from build123d import *
from OCP.BRepFilletAPI import BRepFilletAPI_MakeFillet

# Parameters (mm, degrees)
SKETCH1_W              = 119.42
SKETCH1_H              = 25.4
BOSS_EXTRUDE1_DEPTH    = 3.175
SKETCH2_R              = 3.175
SKETCH2_W              = 25.4
SKETCH2_H              = 3.175
BOSS_EXTRUDE3_DEPTH    = 3.175
FILLET2_R              = 5
FILLET2_R_2            = 4
FILLET2_OF_MIRROR3_R   = 5
FILLET2_OF_MIRROR3_R_2 = 4
FILLET3_R              = 5
SKETCH3_R              = 4.425
CUT_EXTRUDE1_DEPTH     = 10
BOSS_EXTRUDE4_DEPTH    = 3.175
SKETCH9_W              = 55
SKETCH9_H              = 15.875
SKETCH9_R              = 1.5
BOSS_EXTRUDE7_DEPTH    = 3.175
BOSS_EXTRUDE8_DEPTH    = 3.175
FILLET4_R              = 5
SKETCH11_W             = 7.5
SKETCH11_H             = 3.175
BOSS_EXTRUDE9_DEPTH    = 13
SKETCH12_R             = 2.5
CUT_EXTRUDE2_DEPTH     = 10


with BuildPart() as part:
    # Sketch1 → Boss-Extrude1 (new body)
    with BuildSketch(Plane(origin=(0, 0, 0), x_dir=(1, 0, 0), z_dir=(0, 1, 0))):
        Rectangle(SKETCH1_W, SKETCH1_H)
    extrude(amount=BOSS_EXTRUDE1_DEPTH)

    # Sketch2 → Boss-Extrude3 (add)
    # profile 1 of 2: a face of its own
    with BuildSketch(Plane(origin=(59.71, 0, 0), x_dir=(0, 0, -1), z_dir=(1, 0, 0))):
        Polygon((-12.7, 12.3), (-12.7, 3.175), (12.7, 3.175), (12.7, 12.3), (38.2, 12.3), (43.2, 12.3), (43.2, 25), (38.2, 25), (12.7, 25), (-12.7, 25), (-17.7, 25), (-17.7, 12.3), align=None)
        with Locations((-12.7, 18.65)):
            Circle(SKETCH2_R, mode=Mode.SUBTRACT)
        with Locations((38.2, 18.65)):
            Circle(SKETCH2_R, mode=Mode.SUBTRACT)
    # profile 2 of 2: a face of its own
    with BuildSketch(Plane(origin=(59.71, 0, 0), x_dir=(0, 0, -1), z_dir=(1, 0, 0))):
        with Locations((0, 1.5875)):
            Rectangle(SKETCH2_W, SKETCH2_H)
    boss_extrude3 = extrude(amount=-BOSS_EXTRUDE3_DEPTH)

    # Fillet2
    fillet2_edges_1 = [part.edges().sort_by_distance(p)[0] for p in [
        (58.1225, 25, -43.2),
        (58.1225, 12.3, -43.2),
        (58.1225, 12.3, 17.7),
        (58.1225, 25, 17.7),
    ]]
    fillet2_edges_2 = [part.edges().sort_by_distance(p)[0] for p in [
        (58.1225, 12.3, -12.7),
    ]]
    fillet2 = BRepFilletAPI_MakeFillet(part.part.solid().wrapped)
    for e in fillet2_edges_1:
        fillet2.Add(FILLET2_R - 0.0001, e.wrapped)
    for e in fillet2_edges_2:
        fillet2.Add(FILLET2_R_2 - 0.0001, e.wrapped)
    add(Compound.cast(fillet2.Shape()), mode=Mode.REPLACE)  # a hair under: the kernel refuses the full size

    # Mirror3: Boss-Extrude3 across plane
    add(boss_extrude3.mirror(Plane(origin=(0, 0, 0), x_dir=(0, 0, 1), z_dir=(1, 0, 0))))

    # Fillet2 of Mirror3
    fillet2_of_mirror3_edges_1 = [part.edges().sort_by_distance(p)[0] for p in [
        (-58.1225, 25, -43.2),
        (-58.1225, 12.3, -43.2),
        (-58.1225, 12.3, 17.7),
        (-58.1225, 25, 17.7),
    ]]
    fillet2_of_mirror3_edges_2 = [part.edges().sort_by_distance(p)[0] for p in [
        (-58.1225, 12.3, -12.7),
    ]]
    fillet2_of_mirror3 = BRepFilletAPI_MakeFillet(part.part.solid().wrapped)
    for e in fillet2_of_mirror3_edges_1:
        fillet2_of_mirror3.Add(FILLET2_OF_MIRROR3_R - 0.0001, e.wrapped)
    for e in fillet2_of_mirror3_edges_2:
        fillet2_of_mirror3.Add(FILLET2_OF_MIRROR3_R_2 - 0.0001, e.wrapped)
    add(Compound.cast(fillet2_of_mirror3.Shape()), mode=Mode.REPLACE)  # a hair under: the kernel refuses the full size

    # Fillet3
    fillet3_edges = [part.edges().sort_by_distance(p)[0] for p in [
        (56.535, 3.175, 0),
        (59.71, 0, 0),
        (-59.71, 0, 0),
        (-56.535, 3.175, 0),
    ]]
    fillet(fillet3_edges, radius=FILLET3_R)

    # Sketch3 → Cut-Extrude1 (cut)
    with BuildSketch(Plane(origin=(0, 3.175, 0), x_dir=(1, 0, 0), z_dir=(0, 1, 0))):
        with Locations(Location((-15, 0, 0), (0, 0, 270))):
            Circle(SKETCH3_R)
        with Locations(Location((15, 0, 0), (0, 0, 270))):
            Circle(SKETCH3_R)
    extrude(amount=-CUT_EXTRUDE1_DEPTH, mode=Mode.SUBTRACT)

    # Sketch4 → Boss-Extrude4 (add)
    with BuildSketch(Plane(origin=(0, 3.175, 0), x_dir=(1, 0, 0), z_dir=(0, 1, 0))):
        Polygon((-12.5, 60), (12.5, 60), (12.5, 12.7), (6.15, 12.7), (6.15, 19.05), (6.15, 56.825), (-6.15, 56.825), (-6.15, 22.225), (-6.15, 12.7), (-12.5, 12.7), align=None)
    extrude(amount=-BOSS_EXTRUDE4_DEPTH)

    # Sketch9 → Boss-Extrude7 (add)
    with BuildSketch(Plane(origin=(0, 0, -60), x_dir=(-1, 0, 0), z_dir=(0, 0, -1))):
        with Locations((0, -4.7625)):
            Rectangle(SKETCH9_W, SKETCH9_H)
        with Locations((-20, -6.35)):
            Circle(SKETCH9_R, mode=Mode.SUBTRACT)
        with Locations((20, -6.35)):
            Circle(SKETCH9_R, mode=Mode.SUBTRACT)
    extrude(amount=-BOSS_EXTRUDE7_DEPTH)

    # Sketch10 → Boss-Extrude8 (add)
    with BuildSketch(Plane(origin=(27.5, 0, 0), x_dir=(0, 0, -1), z_dir=(1, 0, 0))):
        Polygon((56.825, -12.7), (12.7, 0), (12.7, 3.175), (60, 3.175), (60, -12.7), align=None)
    boss_extrude8 = extrude(amount=BOSS_EXTRUDE8_DEPTH)

    # Mirror4: Boss-Extrude8 across plane
    add(boss_extrude8.mirror(Plane(origin=(0, 0, 0), x_dir=(0, 0, 1), z_dir=(1, 0, 0))))

    # Fillet4
    fillet4_edges = [part.edges().sort_by_distance(p)[0] for p in [
        (12.5, 1.5875, -12.7),
        (6.15, 1.5875, -12.7),
        (-6.15, 1.5875, -12.7),
        (-12.5, 1.5875, -12.7),
        (27.5, 1.5875, -12.7),
        (30.675, 1.5875, -12.7),
        (-30.675, 1.5875, -12.7),
        (-27.5, 1.5875, -12.7),
    ]]
    fillet(fillet4_edges, radius=FILLET4_R)

    # Sketch11 → Boss-Extrude9 (add)
    with BuildSketch(Plane(origin=(0, 3.175, 0), x_dir=(1, 0, 0), z_dir=(0, 1, 0))):
        with Locations((47.785, 11.1125)):
            Rectangle(SKETCH11_W, SKETCH11_H)
        with Locations((9.785, 11.1125)):
            Rectangle(SKETCH11_W, SKETCH11_H)
    extrude(amount=BOSS_EXTRUDE9_DEPTH)

    # Sketch12 → Cut-Extrude2 (cut)
    with BuildSketch(Plane.XY.offset(-9.525)):
        with Locations((9.785, 9.675)):
            Circle(SKETCH12_R)
        with Locations((47.785, 9.675)):
            Circle(SKETCH12_R)
    extrude(amount=-CUT_EXTRUDE2_DEPTH, mode=Mode.SUBTRACT)


solid = part.part
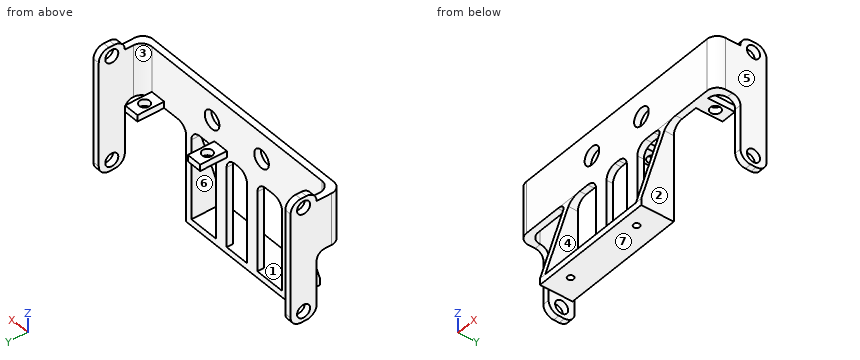
For this review, take the finished solid that the model builds, in its own axes (mm). Face numbers are marked on the shaded views. A direction names the side the tool comes from. Round coordinates to 2 decimals unless told otherwise and drop trailing zeros. Loops run counter-clockwise (first coordinate to the right, second up) from the corner with the lowest first, then second, coordinate; pieces in that order, holes last. Notation, with made-up numbers: (62.25, -39.5) - (86.25, -39.5) arc R15 ccw to (86.25, -11.5) - close; hole circle Ø4 at (12.25, -25). An arc over 180 degrees is marked (long way). Put each result on its own line as item: value. Start each with the question number.
1. For probe 1 along X at (y, z) = (17, -8) (3 decimals); probe 2 along Y at (x, z) = (-57.2, -38.2) (3 decimals); probe 3 along Y at (x, z) = (-20, -58.35) (3 decimals), list the stretches that pass through material, from the lowest coordinate up. Write a range as [from, to].
2. Consider section C-C on z = -54.5. State the section outline as (x, y) points (3 decimals).
3. Mouldability with a two-part tool opening along X and no side actions: class the marked faces 5, 6 and 7 as +X half, -X half, draft (parallel to the pull), parting line (faces both ways), or undercut.
4. For the marked faces 1, 2, 3 and 4, list the 3-axis set-ups (+Z, -Z, +X, -X, +Y, -Y) from which the entire face can be reached by the end or side of a thin tool; tool diameter is ignored.
5. Insertion check: P1, Ø2, axis at x = 58, y = 19, coming from the -Z side; P2, Ø10, axis at x = 14.5, y = 20, coming from the -Z side; P3, Ø3.5, axis at y = 2, z = -46, coming from the -X side (3 decimals); P4, Ø8, axis at y = 7.5, z = -25.5, coming from the +X side. Each pin has a flat end and moves straight along its axis. Give the tip position at first contact, or say it passes through.
6. Consider section B-B on y = 18.65. State the section outline as (x, z) points (3 decimals).
7. Consider section D-D on x = 8.5. State the section outline as (y, z) points (3 decimals).
8. Consider section A-A on z = 0. State the section outline as (x, y) points (3 decimals).
Result sheet:
1. probe 1: [-59.71, -56.535], [56.535, 59.71]
1. probe 2: [12.3, 15.475], [21.825, 25]
1. probe 3: [-12.7, -7.85], [-4.85, 3.175]
2. outline: (-30.675, -12.031) - (-27.5, -12.031) - (-27.5, 3.175) - (-30.675, 3.175) - close; (-12.5, 0) - (-6.15, 0) - (-6.15, 3.175) - (-12.5, 3.175) - close; (6.15, 0) - (12.5, 0) - (12.5, 3.175) - (6.15, 3.175) - close; (27.5, -12.031) - (30.675, -12.031) - (30.675, 3.175) - (27.5, 3.175) - close
3. face 5: +X half
3. face 6: undercut
3. face 7: draft
4. face 1: -Y
4. face 2: -Z, +X, +Y, -Y
4. face 3: +Z, -Z, +Y
4. face 4: +Y, -Y
5. P1: z = -43.2
5. P2: z = -12.7
5. P3: x = -30.675
5. P4: through
6. outline: (-59.71, -43.2) - (-56.535, -43.2) - (-56.535, -41.375) - (-59.71, -41.375) - close; (-59.71, -35.025) - (-56.535, -35.025) - (-56.535, 9.525) - (-59.71, 9.525) - close; (-59.71, 15.875) - (-56.535, 15.875) - (-56.535, 17.7) - (-59.71, 17.7) - close; (56.535, -43.2) - (59.71, -43.2) - (59.71, -41.375) - (56.535, -41.375) - close; (56.535, -35.025) - (59.71, -35.025) - (59.71, 9.525) - (56.535, 9.525) - close; (56.535, 15.875) - (59.71, 15.875) - (59.71, 17.7) - (56.535, 17.7) - close
7. outline: (-12.7, -60) - (3.175, -60) - (3.175, -12.7) - (7.531, -12.7) - (7.531, -9.525) - (3.175, -9.525) - (3.175, 12.7) - (0, 12.7) - (0, -56.825) - (-12.7, -56.825) - close; (11.819, -12.7) - (16.175, -12.7) - (16.175, -9.525) - (11.819, -9.525) - close
8. outline: (-59.71, 5) arc R5 ccw to (-54.71, 0) - (-19.425, 0) - (-19.425, 3.175) - (-51.535, 3.175) arc R5 cw to (-56.535, 8.175) - (-56.535, 25) - (-59.71, 25) - close; (-10.575, 0) - (10.575, 0) - (10.575, 3.175) - (-10.575, 3.175) - close; (19.425, 0) - (54.71, 0) arc R5 ccw to (59.71, 5) - (59.71, 25) - (56.535, 25) - (56.535, 8.175) arc R5 cw to (51.535, 3.175) - (19.425, 3.175) - close
